Read the model definition and answer for the solid it produces. Units are mm, in the model's axes. A direction names the side the tool comes from. Coordinates: 2 decimals unless noted, no trailing zeros. Order: outer loops, then holes, each group sorted by start corner. A loop starts at its lowest first (then second) coordinate and runs counter-clockwise, first axis right, second up. Notation, with made-up numbers: (-30, 28) -> (-11, 28) arc R36 ccw to (-11, 66) -> close; hole circle Ø1 at (47, 65.25). An arc over 180 degrees is marked (long way). Use CSV: the item, a comma, the result in double quotes.
```python
from build123d import *

# Parameters (mm, degrees)
BOSS_EXTRUDE1_DEPTH     = 7
BOSS_EXTRUDE2_DEPTH     = 7
SKETCH4_R               = 4
CUT_EXTRUDE1_DEPTH      = 47.435908473
CUT_EXTRUDE1_DEPTH_BACK = 14


with BuildPart() as part:
    # Sketch1 → Boss-Extrude1 (new body)
    with BuildSketch(Plane(origin=(0, 0, 0), x_dir=(1, 0, 0), z_dir=(0, 1, 0))):
        Polygon((-44, 25), (-38, 31), (38, 31), (44, 25), (44, -25), (38, -31), (-38, -31), (-44, -25), align=None)
        with BuildLine():
            Line((-36, -20.5), (-36, 20.5))
            ThreePointArc((-36, 20.5), (-33, 23.5), (-30, 20.5))
            Line((-30, 20.5), (-30, -20.5))
            ThreePointArc((-30, -20.5), (-33, -23.5), (-36, -20.5))
        make_face(mode=Mode.SUBTRACT)
        with BuildLine():
            Line((36, -20.5), (36, 20.5))
            ThreePointArc((36, 20.5), (33, 23.5), (30, 20.5))
            Line((30, 20.5), (30, -20.5))
            ThreePointArc((30, -20.5), (33, -23.5), (36, -20.5))
        make_face(mode=Mode.SUBTRACT)
    extrude(amount=BOSS_EXTRUDE1_DEPTH)

    # Sketch3 → Boss-Extrude2 (add, symmetric)
    with BuildSketch(Plane(origin=(0, 0, 0), x_dir=(0.849441251, 0, -0.527683201), z_dir=(0.527683201, 0, 0.849441251))):
        Polygon((15.483777963, 7), (-18.849066913, 7), (25.26789187, 39.052846762), (27.619032879, 35.816778784), (15.483777963, 27), align=None)
    extrude(amount=BOSS_EXTRUDE2_DEPTH, both=True)

    # Sketch4 → Cut-Extrude1 (cut, two sides)
    with BuildSketch(Plane(origin=(-8.359258135, 13.544823437, 5.192872478), x_dir=(0.866435488, 0.466201263, 0.178734239), z_dir=(-0.49928904, 0.809016994, 0.310164404))) as cut_extrude1_sk:
        with Locations((28.868116916, 22.166684098)):
            Circle(SKETCH4_R)
        with BuildLine():
            ThreePointArc((24.604923104, 27.718726833), (29.779470735, 29.107104418), (34.420159658, 26.4298779))
            Line((34.420159658, 26.4298779), (30.156965838, 31.981920644))
            Line((30.156965838, 31.981920644), (24.604923104, 27.718726833))
        make_face()
        with BuildLine():
            ThreePointArc((34.420159658, 26.4298779), (35.808537235, 21.255330279), (33.131310727, 16.614641364))
            Line((33.131310727, 16.614641364), (38.683353462, 20.877835176))
            Line((38.683353462, 20.877835176), (34.420159658, 26.4298779))
        make_face()
    extrude(amount=CUT_EXTRUDE1_DEPTH, mode=Mode.SUBTRACT)
    extrude(cut_extrude1_sk.sketch, amount=-CUT_EXTRUDE1_DEPTH_BACK, mode=Mode.SUBTRACT)


solid = part.part
```
Item 1: Find section D-D, the plane x = -15.5. Give the vertices of the cut face in (y, z).
Return value:
outline,"(0, -31) -> (7, -31) -> (7, 1.39) -> (10.6, 1.39) -> (7, 10.77) -> (7, 31) -> (0, 31) -> close"
Item 2: Find section C-C, the plane y = 5.5. Give the vertices of the cut face in (x, z).
Return value:
outline,"(-44, -25) -> (-38, -31) -> (38, -31) -> (44, -25) -> (44, 25) -> (38, 31) -> (-38, 31) -> (-44, 25) -> close; hole (-36, -20.5) arc R3 ccw to (-30, -20.5) -> (-30, 20.5) arc R3 ccw to (-36, 20.5) -> close; hole (30, -20.5) arc R3 ccw to (36, -20.5) -> (36, 20.5) arc R3 ccw to (30, 20.5) -> close"
Item 3: The mould has two halves that part along Z. Classify faces 1 (the flat face through (1.72, 18.06, -9.31)), 2 (the cylindrical face through (33.1, 3.5, -23.5)), 3 (the flat face through (10, 7, 6)): +Z half, -Z half, draft (parallel to the pull), parting line (faces both ways), or undercut.
Return value:
face 1,"-Z half"
face 2,"undercut"
face 3,"draft"
Item 4: Find section B-B, the plane z = -19.5. Give the vertices of the cut face in (x, y).
Return value:
outline,"(-44, 0) -> (-36, 0) -> (-36, 7) -> (-44, 7) -> close; (-30, 0) -> (30, 0) -> (30, 7) -> (-30, 7) -> close; (36, 0) -> (44, 0) -> (44, 7) -> (36, 7) -> close"
Item 5: Straight lines are drawn through the part: line 1 along Y through (x, z) = (-24.5, 26.5); line 2 along X through (y, z) = (10.5, 9); line 3 along X through (y, z) = (32, -12.5). For each, find the intervals that lie inside material, in ascending order.
Return value:
line 1,"y = 0 to 7"
line 2,"x = -10.93 to -1.22"
line 3,"x = 10.55 to 14.2"
Item 6: Each of these flat-tipped pins is pushed along its axis until it touches: P1, Ø2, axis at x = 6.5, z = 9, coming from the +Y side; P2, Ø4, axis at y = 23.5, z = -11, coming from the -X side; P3, Ø5, axis at x = 6.5, z = -4.5, coming from the +Y side; P4, Ø1, axis at x = 4, z = -20, coming from the -Y side. Where does it stop, or does it pass through?
Return value:
P1,"stops at y = 7"
P2,"stops at x = 1.22"
P3,"stops at y = 28.25"
P4,"stops at y = 0"
Item 7: Find section A-A, the plane x = -33. Give the vertices of the cut face in (y, z).
Return value:
outline,"(0, -31) -> (7, -31) -> (7, -23.5) -> (0, -23.5) -> close; (0, 23.5) -> (7, 23.5) -> (7, 31) -> (0, 31) -> close"
Item 8: A tool of negligible diameter and unlimited length cuts with its end or side. For faces 4 (the cylindrical face through (32.9, 3.5, 23.5)), 5 (the flat face through (9.11, 18.06, 2.58)), 6 (the flat face through (13.204, 17.14, -8.087)), from which of +Z, -Z, +X, -X, +Y, -Y can it reach the whole face along a straight path? Write none if from no direction.
Return value:
face 4,"+Y, -Y"
face 5,"+Z, +X, +Y"
face 6,"-Z, +X"
